The model under review builds one solid part; all positions refer to its coordinate system, in mm. A direction names the side the tool comes from. Give positions to 0.01 mm unless a question says otherwise; leave off trailing zeros. Loops run counter-clockwise (first coordinate to the right, second up) from the corner with the lowest first, then second, coordinate; pieces in that order, holes last. Notation, with made-up numbers: (88.25, 67) - (146.25, 67) arc R15 cw to (146.25, 85) - close; hole circle Ø4 at (-38, -15). An arc over 180 degrees is marked (long way). Return JSON: item names as keys, results as strings. Group by question number.
```python
from build123d import *

# Parameters (mm, degrees)
BOSS_EXTRUDE1_DEPTH              = 76.2
CUT_EXTRUDE3_DEPTH               = 47.625
CUT_EXTRUDE4_DEPTH               = 110.433918417
F_10_0_1935_DIAMETER_HOLE1_D     = 4.9149
F_10_0_1935_DIAMETER_HOLE1_DEPTH = 19.05
F_10_0_1935_DIAMETER_HOLE1_TIP   = 1.476584928
F_1_4_20_TAPPED_HOLE1_D          = 5.1054
SKETCH19_R                       = 2.499999953
CUT_EXTRUDE5_DEPTH               = 87.135590889
F_1_4_20_TAPPED_HOLE2_D          = 5.1054
F_1_4_20_TAPPED_HOLE2_DEPTH      = 20.691183098
F_1_4_20_TAPPED_HOLE2_TIP        = 1.533816902
F_1_4_20_TAPPED_HOLE3_D          = 5.1054
F_1_4_20_TAPPED_HOLE3_DEPTH      = 9.05002
F_1_4_20_TAPPED_HOLE3_TIP        = 1.533816902
F_1_4_20_TAPPED_HOLE4_D          = 5.1054
F_1_4_20_TAPPED_HOLE4_DEPTH      = 7.356183098
F_1_4_20_TAPPED_HOLE4_TIP        = 1.533816902


with BuildPart() as part:
    # Sketch1 → Boss-Extrude1 (new, symmetric)
    with BuildSketch(Plane(origin=(0, 0, 0), x_dir=(1, 0, 0), z_dir=(0, 1, 0))):
        Polygon((-15.875, 6.35), (-15.875, 19.05), (15.875, 19.05), (15.875, 6.35), (38.1, 6.35), (38.1, -6.35), (-38.1, -6.35), (-38.1, 6.35), align=None)
    extrude(amount=BOSS_EXTRUDE1_DEPTH, both=True)

    # Sketch5 → Cut-Extrude3 (cut, symmetric)
    with BuildSketch(Plane(origin=(0, 0, 0), x_dir=(1, 0, 0), z_dir=(0, 1, 0))):
        with BuildLine():
            Line((-4.7625, 19.05), (-4.7625, 12.7))
            ThreePointArc((-4.7625, 12.7), (0, 7.9375), (4.7625, 12.7))
            Line((4.7625, 12.7), (4.7625, 19.05))
            Line((4.7625, 19.05), (-4.7625, 19.05))
        make_face()
    extrude(amount=CUT_EXTRUDE3_DEPTH, both=True, mode=Mode.SUBTRACT)

    # Sketch9 → Cut-Revolve1 (revolve, cut)
    with BuildSketch(Plane(origin=(0, 0, 0), x_dir=(0, 0, -1), z_dir=(1, 0, 0))):
        with BuildLine():
            Line((19.05, -52.3875), (12.7, -52.3875))
            ThreePointArc((12.7, -52.3875), (9.332403955, -50.992596045), (7.9375, -47.625))
            Line((7.9375, -47.625), (19.05, -47.625))
            Line((19.05, -47.625), (19.05, -52.3875))
        make_face()
    cut_revolve1 = revolve(axis=Axis((0, -47.625, -7.9375), (0, 0, -1)), mode=Mode.SUBTRACT)

    # Mirror1: Cut-Revolve1 across plane
    add(cut_revolve1.mirror(Plane.ZX), mode=Mode.SUBTRACT)

    # Sketch12 → Cut-Extrude4 (cut, through all)
    with BuildSketch(Plane(origin=(38.1, 0, 0), x_dir=(0, 0, -1), z_dir=(1, 0, 0))):
        Polygon((-6.35, -63.5), (0, -63.5), (0, -44.45), (1.5875, -33.956087115), (1.5875, -4.143912885), (0, 6.35), (0, 19.05), (-6.35, 19.05), align=None)
    extrude(amount=-CUT_EXTRUDE4_DEPTH, mode=Mode.SUBTRACT)

    # #10 (0.1935) Diameter Hole1
    with Locations(Plane(origin=(0, -76.2, 0), x_dir=(-1, 0, 0), z_dir=(0, -1, 0))):
        with Locations((25.4, -3.175), (-25.4, -3.175), (0, -3.175)):
            Hole(F_10_0_1935_DIAMETER_HOLE1_D / 2, depth=F_10_0_1935_DIAMETER_HOLE1_DEPTH)
            with Locations((0, 0, -(F_10_0_1935_DIAMETER_HOLE1_DEPTH + F_10_0_1935_DIAMETER_HOLE1_TIP / 2))):  # 118° drill point
                Cone(0, F_10_0_1935_DIAMETER_HOLE1_D / 2, F_10_0_1935_DIAMETER_HOLE1_TIP, mode=Mode.SUBTRACT)

    # 1/4-20 Tapped Hole1 (through all)
    with Locations(Plane(origin=(0, 76.2, 0), x_dir=(1, 0, 0), z_dir=(0, 1, 0))):
        with Locations((0, 12.7)):
            Hole(F_1_4_20_TAPPED_HOLE1_D / 2)

    # Sketch19 → Cut-Extrude5 (cut, through all)
    with BuildSketch(Plane(origin=(0, 0, -6.35), x_dir=(-1, 0, 0), z_dir=(0, 0, -1))):
        with Locations((-27.209019229, 44.45)):
            Circle(SKETCH19_R)
    extrude(amount=-CUT_EXTRUDE5_DEPTH, mode=Mode.SUBTRACT)

    # 1/4-20 Tapped Hole2
    with Locations(Plane(origin=(0, 76.2, 0), x_dir=(1, 0, 0), z_dir=(0, 1, 0))):
        with Locations((27.94, 0), (-27.94, 0)):
            Hole(F_1_4_20_TAPPED_HOLE2_D / 2, depth=F_1_4_20_TAPPED_HOLE2_DEPTH)
            with Locations((0, 0, -(F_1_4_20_TAPPED_HOLE2_DEPTH + F_1_4_20_TAPPED_HOLE2_TIP / 2))):  # 118° drill point
                Cone(0, F_1_4_20_TAPPED_HOLE2_D / 2, F_1_4_20_TAPPED_HOLE2_TIP, mode=Mode.SUBTRACT)

    # 1/4-20 Tapped Hole3
    with Locations(Plane(origin=(0, 0, -19.05), x_dir=(-1, 0, 0), z_dir=(0, 0, -1))):
        with Locations((-9.525, -66.675), (9.525, 57.15), (-9.525, 57.15), (9.525, -66.675)):
            Hole(F_1_4_20_TAPPED_HOLE3_D / 2, depth=F_1_4_20_TAPPED_HOLE3_DEPTH)
            with Locations((0, 0, -(F_1_4_20_TAPPED_HOLE3_DEPTH + F_1_4_20_TAPPED_HOLE3_TIP / 2))):  # 118° drill point
                Cone(0, F_1_4_20_TAPPED_HOLE3_D / 2, F_1_4_20_TAPPED_HOLE3_TIP, mode=Mode.SUBTRACT)

    # 1/4-20 Tapped Hole4
    with Locations(Plane.XY.offset(6.35)):
        with Locations((19.05, 30.260695081), (-19.05, 30.260695081)):
            Hole(F_1_4_20_TAPPED_HOLE4_D / 2, depth=F_1_4_20_TAPPED_HOLE4_DEPTH)
            with Locations((0, 0, -(F_1_4_20_TAPPED_HOLE4_DEPTH + F_1_4_20_TAPPED_HOLE4_TIP / 2))):  # 118° drill point
                Cone(0, F_1_4_20_TAPPED_HOLE4_D / 2, F_1_4_20_TAPPED_HOLE4_TIP, mode=Mode.SUBTRACT)


solid = part.part
```
1) For pin 1 Ø11 at (x, y) = (-23, -12.5) entering from -Z; pin 2 Ø14 at (y, z) = (-18.5, -14) entering from -X (3 decimals); pin 3 Ø5 at (y, z) = (-21.5, -15.5) entering from +X (3 decimals), all flat-tipped, find the tip position at first contact; note any pin that passes through.
2) We need section D-D, the plane x = 32. Write out the cut boundary in (y, z).
3) To check wall thickness, follow line 1 (Y direction, x = 34.5, z = 0.5); line 2 (X direction, y = 52.5, z = -13.25) (3 decimals); line 3 (Z direction, x = -27.5, y = -56). State the ranges of each line that lie inside material, in increasing order.
4) We need section C-C, the plane y = 62.5. Write out the cut boundary in (x, z) (3 decimals).
5) Draft analysis for pull direction Y (two halves, no side actions). For faces 6 (the face through (-38.1, 18, -1)), 7 (the face through (28.35, 54.24, 0.17)), 8 (the face through (1, 13, 0)), state which applies: +Y half, -Y half, draft (parallel to the pull), parting line (faces both ways), or undercut.
6) Tool access review of faces 1 (the face through (0.533, 1.03, -0.805)), 2 (the face through (-27, 1, -6.35)), 3 (the face through (30.49, 65.71, -0.11)), 4 (the face through (0.105, -52.386, -15.831)), 5 (the face through (16.692, 29.283, 2.62)): name each direction out of +Z, -Z, +X, -X, +Y, -Y from which nothing blocks a thin tool from reaching the whole face with its end or side.
7) We need section B-B, the plane x = 0. Count the separate pieces of the cut face and the enclosed holes in it, plus the area to 3 significant figures.
Findings:
{
 "1": {"pin 1": "stops at z = -6.35", "pin 2": "stops at x = -15.875", "pin 3": "stops at x = 15.875"},
 "2": {"outline": "(-76.2, -6.35) - (76.2, -6.35) - (76.2, 6.35) - (19.05, 6.35) - (19.05, 0) - (6.35, 0) - (-4.14, -1.59) - (-33.96, -1.59) - (-44.45, 0) - (-63.5, 0) - (-63.5, 6.35) - (-76.2, 6.35) - close"},
 "3": {"line 1": "y = -76.2 to -63.5, 19.05 to 76.2", "line 2": "x = -15.875 to -2.493, 2.493 to 15.875", "line 3": "z = -6.35 to 0"},
 "4": {"outline": "(-38.1, -6.35) - (-15.875, -6.35) - (-15.875, -19.05) - (15.875, -19.05) - (15.875, -6.35) - (38.1, -6.35) - (38.1, 6.35) - (-38.1, 6.35) - close; hole circle Ø5.105 at (-27.94, 0); hole circle Ø5.105 at (0, -12.7); hole circle Ø5.105 at (27.94, 0)"},
 "5": {"face 6": "draft", "face 7": "+Y half", "face 8": "undercut"},
 "6": {"face 1": "+Z, +X, -X", "face 2": "-Z, -X, +Y, -Y", "face 3": "+Y", "face 4": "-Z", "face 5": "+Z"},
 "7": {"separate pieces": "4", "enclosed holes": "0", "area": "1,820 mm^2"}
}
